Check sheet for the modelled part. Datum: model origin and axes. Units: mm. A direction names the side the tool comes from. Give positions to 0.01 mm unless a question says otherwise; leave off trailing zeros. Order: outer loops, then holes, each group sorted by start corner. A loop starts at its lowest first (then second) coordinate and runs counter-clockwise, first axis right, second up. Notation, with made-up numbers: (12.5, 9.25) - (62.5, 9.25) arc R10 cw to (62.5, 17.25) - close; hole circle Ø9 at (59, -11.75). An arc over 180 degrees is marked (long way). Answer in a Markdown table with one row per item.
from build123d import *

# Parameters (mm, degrees)
ESBO_O1_W                = 220
ESBO_O1_H                = 60
ESBO_O1_R                = 4
ESBO_O1_W_2              = 42.3
ESBO_O1_H_2              = 42.3
RESSALTO_EXTRUS_O1_DEPTH = 5
CHANFRO1_SIZE            = 5.6002
ESBO_O2_R                = 8
ESBO_O2_R_2              = 4
RESSALTO_EXTRUS_O2_DEPTH = 10
ESBO_O3_R                = 1.75
CORTE_EXTRUS_O1_DEPTH    = 10
FILETE1_R                = 2


with BuildPart() as part:
    # Esboço1 → Ressalto-extrusão1 (new body, symmetric)
    with BuildSketch(Plane.XY):
        Rectangle(ESBO_O1_W, ESBO_O1_H)
        with Locations((100, 0)):
            Circle(ESBO_O1_R, mode=Mode.SUBTRACT)
        with Locations((-100, 0)):
            Circle(ESBO_O1_R, mode=Mode.SUBTRACT)
        Rectangle(ESBO_O1_W_2, ESBO_O1_H_2, mode=Mode.SUBTRACT)
    extrude(amount=RESSALTO_EXTRUS_O1_DEPTH, both=True)

    # Chanfro1
    chanfro1_edges = [part.edges().sort_by_distance(p)[0] for p in [
        (21.15, -21.15, 0),
        (21.15, 21.15, 0),
        (-21.15, 21.15, 0),
        (-21.15, -21.15, 0),
    ]]
    chamfer(chanfro1_edges, length=CHANFRO1_SIZE)

    # Esboço2 → Ressalto-extrusão2 (add)
    with BuildSketch(Plane.XY.offset(5)):
        with Locations((-100, 0)):
            Circle(ESBO_O2_R)
        with Locations((-100, 0)):
            Circle(ESBO_O2_R_2, mode=Mode.SUBTRACT)
        with Locations((100, 0)):
            Circle(ESBO_O2_R)
        with Locations((100, 0)):
            Circle(ESBO_O2_R_2, mode=Mode.SUBTRACT)
    extrude(amount=RESSALTO_EXTRUS_O2_DEPTH)

    # Esboço3 → Corte-extrusão1 (cut)
    with BuildSketch(Plane.XY.offset(5)):
        with Locations((-30, 25)):
            Circle(ESBO_O3_R)
        with Locations((-30, -25)):
            Circle(ESBO_O3_R)
        with Locations((30, 25)):
            Circle(ESBO_O3_R)
        with Locations((30, -25)):
            Circle(ESBO_O3_R)
    extrude(amount=-CORTE_EXTRUS_O1_DEPTH, mode=Mode.SUBTRACT)

    # Filete1
    filete1_edges = [part.edges().sort_by_distance(p)[0] for p in [
        (110, -30, 0),
        (-110, -30, 0),
        (-110, 30, 0),
        (110, 30, 0),
    ]]
    fillet(filete1_edges, radius=FILETE1_R)


solid = part.part
(1) Gauge pin test, flat ends, axial feed: P1, Ø7, axis at x = -100, y = 0, coming from the -Z side; P2, Ø6, axis at x = -66.5, y = 16.5, coming from the +Z side; P3, Ø8, axis at y = 7.5, z = 9.5, coming from the +X side. Record the tip position at first contact, or that the pin passes through.
Geometry says:
| item | result |
|---|---|
| P1 | through |
| P2 | z = 5 |
| P3 | x = 107.19 |
(2) Cross-section at C-C, the plane z = 8.5. Record the cut outline in (x, y).
Geometry says:
| item | result |
|---|---|
| outline | circle Ø16 at (-100, 0); circle Ø16 at (100, 0); hole circle Ø8 at (-100, 0); hole circle Ø8 at (100, 0) |
(3) Thickness scan on L1, parallel to Y at x = -30, z = -2; L2, parallel to Y at x = -100, z = 2.25; L3, parallel to X at y = -2.5, z = -1.25. Record the ranges inside material, lowest first.
Geometry says:
| item | result |
|---|---|
| L1 | -30 to -26.75, -23.25 to 23.25, 26.75 to 30 |
| L2 | -30 to -4, 4 to 30 |
| L3 | -110 to -103.12, -96.88 to -21.15, 21.15 to 96.88, 103.12 to 110 |
(4) Cross-section at A-A, the plane x = 100. Record the cut outline in (y, z).
Geometry says:
| item | result |
|---|---|
| outline | (-30, -5) - (-4, -5) - (-4, 15) - (-8, 15) - (-8, 5) - (-30, 5) - close; (4, -5) - (30, -5) - (30, 5) - (8, 5) - (8, 15) - (4, 15) - close |
(5) Cross-section at B-B, the plane y = 13. Record the cut outline in (x, z).
Geometry says:
| item | result |
|---|---|
| outline | (-110, -5) - (-21.15, -5) - (-21.15, 5) - (-110, 5) - close; (21.15, -5) - (110, -5) - (110, 5) - (21.15, 5) - close |
(6) Access from +Z, -Z, +X, -X, +Y, -Y to the whole of each face (thin tool, end or side, straight path). Record for faces 4 (the cylindrical face through (92, 0, 10)), 5 (the flat face through (-2, 30, 0)), 6 (the flat face through (21.15, 0, 0)).
Geometry says:
| item | result |
|---|---|
| face 4 | +Z |
| face 5 | +Z, -Z, +X, -X, +Y |
| face 6 | +Z, -Z |
(7) Mould release check, pull along Y, two halves, no side actions. Record for faces 1 (the flat face through (-2, -30, 0)), 2 (the flat face through (23, 0, 5)), 3 (the flat face through (0, 21.15, 0)): pulls with the +Y half, pulls with the -Y half, needs draft (parallel to the pull), parting line crosses it, or undercut.
Geometry says:
| item | result |
|---|---|
| face 1 | pulls with the -Y half |
| face 2 | needs draft |
| face 3 | undercut |
(8) Cross-section at D-D, the plane x = -79. Record the cut outline in (y, z).
Geometry says:
| item | result |
|---|---|
| outline | (-30, -5) - (30, -5) - (30, 5) - (-30, 5) - close |
